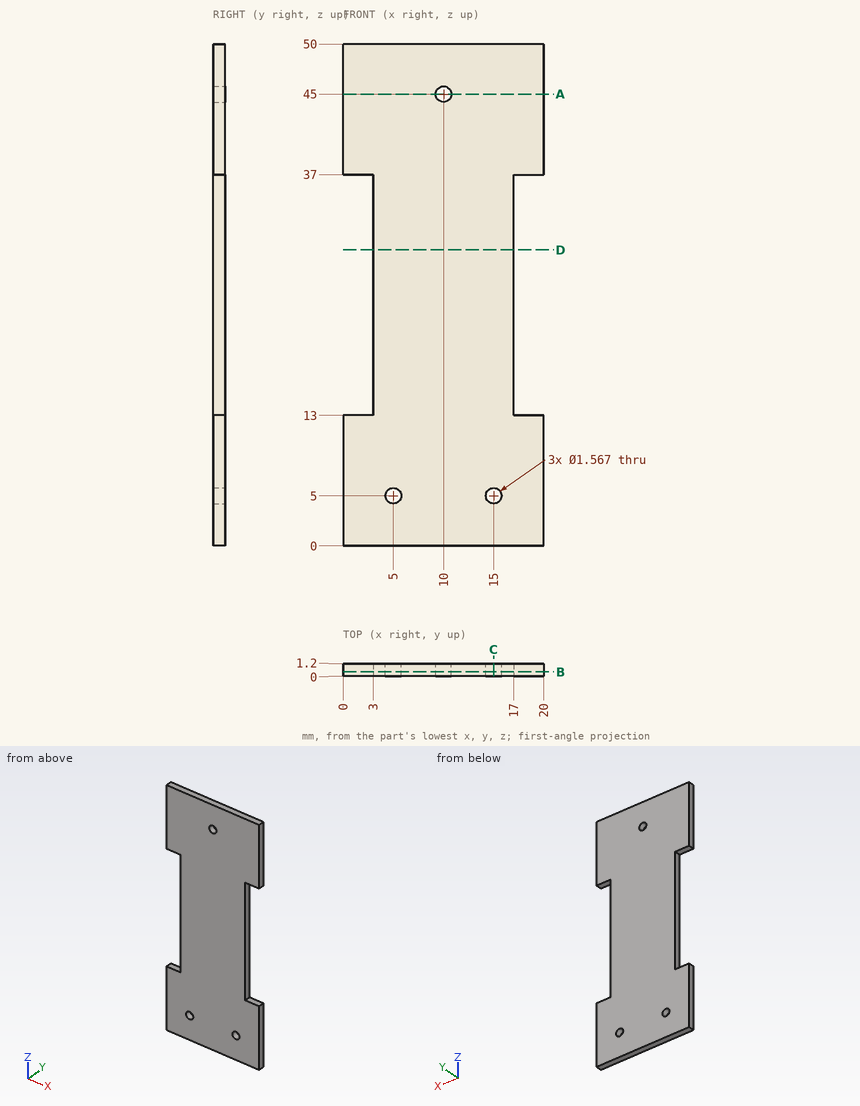
Here's the drawing with two shaded views (mm, measured from the low corner). I have some questions. Coordinates: 2 decimals unless noted, no trailing zeros. Write each loop counter-clockwise with the first axis right and the second up, starting at its lowest first coordinate (ties: lowest second). Pieces come first, ordered by that corner, then holes. Notation, with made-up numbers: (57, 46) -> (113, 46) arc R23 cw to (113, 75) -> close; hole circle Ø3 at (29.25, -29.5). An arc over 180 degrees is marked (long way). Use a Markdown table: item, result. Add a question column.
(1) If we section it at C-C, the plane x = 15: Write out the boundary of the cut face in (y, z), and give its area (3 significant figures).
(2) Please list where these lines run through material, in increasing order: line 1 (X direction, y = 0.3, z = 5); line 2 (Z direction, x = 1.25, y = 1); line 3 (X direction, y = 0.6, z = 45).
(3) If we section it at B-B, the plane y = 0.4: Write out the boundary of the cut face in (x, z).
(4) If we section it at D-D, the plane z = 29.5: Write out the boundary of the cut face in (x, y).
(5) If we section it at A-A, the plane z = 45: Write out the boundary of the cut face in (x, y), and give its area (3 significant figures).
(6) I'm going to push a flat-ended pin straight in: P1, Ø1.4, axis at x = 10, z = 45, coming from the -Y side. Where does the tip first touch, or does it pass through?
Outcome:
| question | item | result |
|---|---|---|
| 1 | outline | (0, 0) -> (1.2, 0) -> (1.2, 4.22) -> (0, 4.22) -> close; (0, 5.78) -> (1.2, 5.78) -> (1.2, 50) -> (0, 50) -> close |
| 1 | area | 58.1 mm^2 |
| 2 | line 1 | x = 0 to 4.22, 5.78 to 14.22, 15.78 to 20 |
| 2 | line 2 | z = 0 to 13, 37 to 50 |
| 2 | line 3 | x = 0 to 9.22, 10.78 to 20 |
| 3 | outline | (0, 0) -> (20, 0) -> (20, 13) -> (17, 13) -> (17, 37) -> (20, 37) -> (20, 50) -> (0, 50) -> (0, 37) -> (3, 37) -> (3, 13) -> (0, 13) -> close; hole circle Ø1.57 at (5, 5); hole circle Ø1.57 at (10, 45); hole circle Ø1.57 at (15, 5) |
| 4 | outline | (3, 0) -> (17, 0) -> (17, 1.2) -> (3, 1.2) -> close |
| 5 | outline | (0, 0) -> (9.22, 0) -> (9.22, 1.2) -> (0, 1.2) -> close; (10.78, 0) -> (20, 0) -> (20, 1.2) -> (10.78, 1.2) -> close |
| 5 | area | 22.1 mm^2 |
| 6 | P1 | passes through |
